The model under review builds one solid part; all positions refer to its coordinate system, in mm. A direction names the side the tool comes from. Coordinates: 2 decimals unless noted, no trailing zeros. Order: outer loops, then holes, each group sorted by start corner. A loop starts at its lowest first (then second) coordinate and runs counter-clockwise, first axis right, second up. Notation, with made-up numbers: (65.25, -32.5) -> (86.25, -32.5) arc R14 cw to (86.25, -26.5) -> close; hole circle Ø2 at (-18, 43). An arc over 180 degrees is marked (long way). Put each result on its own line as item: value.
from build123d import *

# Parameters (mm, degrees)
SKETCH1_W               = 12.7
SKETCH1_H               = 4.064
BOSS_EXTRUDE1_DEPTH     = 228.6
SKETCH2_W               = 3.429
SKETCH2_H               = 217.3732
CUT_EXTRUDE1_DEPTH      = 0.254
SKETCH3_W               = 0.508
SKETCH3_H               = 5.08
CUT_EXTRUDE2_DEPTH      = 229.724285103
MIRROR2_COPY_1_SKETCH_W = 0.508
MIRROR2_COPY_1_SKETCH_H = 5.08
MIRROR2_COPY_1_DEPTH    = 229.724285103
SKETCH4_W               = 3.175
SKETCH4_H               = 3.175
CUT_EXTRUDE3_DEPTH      = 229.724285103
CUT_EXTRUDE5_DEPTH      = 229.724285103
SKETCH6_W               = 6.80212
SKETCH6_H               = 6.80212
SKETCH6_R               = 1.70053
BOSS_EXTRUDE2_DEPTH     = 4.064
FILLET1_R               = 2.54


with BuildPart() as part:
    # Sketch1 → Boss-Extrude1 (new body)
    with BuildSketch(Plane.XY):
        Rectangle(SKETCH1_W, SKETCH1_H)
    extrude(amount=BOSS_EXTRUDE1_DEPTH)

    # Sketch2 → Cut-Extrude1 (cut)
    with BuildSketch(Plane(origin=(0, 2.032, 0), x_dir=(1, 0, 0), z_dir=(0, 1, 0))):
        with Locations((0, -114.3)):
            Rectangle(SKETCH2_W, SKETCH2_H)
    extrude(amount=-CUT_EXTRUDE1_DEPTH, mode=Mode.SUBTRACT)

    # Sketch3 → Cut-Extrude2 (cut, through all)
    with BuildSketch(Plane(origin=(0, 2.032, 0), x_dir=(1, 0, 0), z_dir=(0, 1, 0))):
        with Locations((-6.096, -226.06)):
            Rectangle(SKETCH3_W, SKETCH3_H)
    cut_extrude2 = extrude(amount=-CUT_EXTRUDE2_DEPTH, mode=Mode.SUBTRACT)

    # Mirror1: Cut-Extrude2 across plane
    add(cut_extrude2.mirror(Plane(origin=(0, 0, 114.3), x_dir=(1, 0, 0), z_dir=(0, 0, -1))), mode=Mode.SUBTRACT)

    # Mirror2: Cut-Extrude2 across plane
    add(cut_extrude2.mirror(Plane(origin=(0, 0, 0), x_dir=(0, 0, 1), z_dir=(1, 0, 0))), mode=Mode.SUBTRACT)

    # Mirror2 copy 1 sketch → Mirror2 copy 1 (cut, through all)
    with BuildSketch(Plane(origin=(0, 2.032, 228.6), x_dir=(-1, 0, 0), z_dir=(0, 1, 0))):
        with Locations((-6.096, -226.06)):
            Rectangle(MIRROR2_COPY_1_SKETCH_W, MIRROR2_COPY_1_SKETCH_H)
    extrude(amount=-MIRROR2_COPY_1_DEPTH, mode=Mode.SUBTRACT)

    # Sketch4 → Cut-Extrude3 (cut, through all)
    with BuildSketch(Plane(origin=(0, 2.032, 0), x_dir=(1, 0, 0), z_dir=(0, 1, 0))):
        with Locations((-4.2545, -227.0125)):
            Rectangle(SKETCH4_W, SKETCH4_H)
    extrude(amount=-CUT_EXTRUDE3_DEPTH, mode=Mode.SUBTRACT)

    # Sketch5 → Cut-Extrude5 (cut, through all)
    with BuildSketch(Plane(origin=(0, 2.032, 0), x_dir=(1, 0, 0), z_dir=(0, 1, 0))):
        Polygon((-6.35, -71.12), (-6.35, -152.4), (-6.35, -228.6), (6.35, -228.6), (6.35, -155.575), (6.35, -152.4), (6.35, -76.2), (-3.175, -76.2), (-3.175, -71.12), align=None)
    extrude(amount=-CUT_EXTRUDE5_DEPTH, mode=Mode.SUBTRACT)

    # Sketch6 → Boss-Extrude2 (add, through all)
    # profile 1 of 2: a face of its own
    with BuildSketch(Plane(origin=(0, 2.032, 0), x_dir=(1, 0, 0), z_dir=(0, 1, 0))):
        with Locations((9.75106, -38.1)):
            Rectangle(SKETCH6_W, SKETCH6_H)
        with Locations(Location((9.75106, -38.1, 0), (0, 0, 270))):
            Circle(SKETCH6_R, mode=Mode.SUBTRACT)
    # profile 2 of 2: a face of its own
    with BuildSketch(Plane(origin=(0, 2.032, 0), x_dir=(1, 0, 0), z_dir=(0, 1, 0))):
        with Locations((-9.75106, -38.1)):
            Rectangle(SKETCH6_W, SKETCH6_H)
        with Locations(Location((-9.75106, -38.1, 0), (0, 0, 90))):
            Circle(SKETCH6_R, mode=Mode.SUBTRACT)
    extrude(amount=-BOSS_EXTRUDE2_DEPTH)

    # Fillet1
    fillet1_edges = [part.edges().sort_by_distance(p)[0] for p in [
        (6.35, 0, 41.50106),
        (13.15212, 0, 41.50106),
        (13.15212, 0, 34.69894),
        (6.35, 0, 34.69894),
        (-6.35, 0, 34.69894),
        (-13.15212, 0, 34.69894),
        (-13.15212, 0, 41.50106),
        (-6.35, 0, 41.50106),
    ]]
    fillet(fillet1_edges, radius=FILLET1_R)


solid = part.part
Item 1: Consider section B-B on x = -0.5. Write out the cut boundary in (y, z).
Answers below:
outline: (-2.03, 0) -> (2.03, 0) -> (2.03, 5.61) -> (1.78, 5.61) -> (1.78, 76.2) -> (-2.03, 76.2) -> close
Item 2: Consider section A-A on z = 38.1. Write out the cut boundary in (x, y), and give its area (3 significant figures).
Answers below:
outline: (-13.15, -2.03) -> (-11.45, -2.03) -> (-11.45, 2.03) -> (-13.15, 2.03) -> close; (-8.05, -2.03) -> (8.05, -2.03) -> (8.05, 2.03) -> (1.71, 2.03) -> (1.71, 1.78) -> (-1.71, 1.78) -> (-1.71, 2.03) -> (-8.05, 2.03) -> close; (11.45, -2.03) -> (13.15, -2.03) -> (13.15, 2.03) -> (11.45, 2.03) -> close
area: 78.4 mm^2
Item 3: Consider section D-D on y = 0.45. Write out the cut boundary in (x, z) (3 decimals).
Answers below:
outline: (-13.152, 37.239) arc R2.54 ccw to (-10.612, 34.699) -> (-8.89, 34.699) arc R2.54 cw to (-6.35, 32.159) -> (-6.35, 5.08) -> (-5.842, 5.08) -> (-5.842, 0) -> (5.842, 0) -> (5.842, 5.08) -> (6.35, 5.08) -> (6.35, 32.159) arc R2.54 cw to (8.89, 34.699) -> (10.612, 34.699) arc R2.54 ccw to (13.152, 37.239) -> (13.152, 38.961) arc R2.54 ccw to (10.612, 41.501) -> (8.89, 41.501) arc R2.54 cw to (6.35, 44.041) -> (6.35, 76.2) -> (-3.175, 76.2) -> (-3.175, 71.12) -> (-6.35, 71.12) -> (-6.35, 44.041) arc R2.54 cw to (-8.89, 41.501) -> (-10.612, 41.501) arc R2.54 ccw to (-13.152, 38.961) -> close; hole circle Ø3.401 at (-9.751, 38.1); hole circle Ø3.401 at (9.751, 38.1)
Item 4: Consider section C-C on z = 24.5. Write out the cut boundary in (x, y), and give its area (3 significant figures).
Answers below:
outline: (-6.35, -2.03) -> (6.35, -2.03) -> (6.35, 2.03) -> (1.71, 2.03) -> (1.71, 1.78) -> (-1.71, 1.78) -> (-1.71, 2.03) -> (-6.35, 2.03) -> close
area: 50.7 mm^2
Item 5: For line 1 (X direction, y = 1.25, z = 38.1); line 2 (X direction, y = 1.45, z = 38.5); line 3 (X direction, y = 0.4, z = 49.5), list the stretches that pass through material, from the lowest coordinate up. Write a range as from..to.
Answers below:
line 1: -13.15..-11.45, -8.05..8.05, 11.45..13.15
line 2: -13.15..-11.4, -8.1..8.1, 11.4..13.15
line 3: -6.35..6.35
Item 6: Mouldability with a two-part tool opening along Z and no side actions: class faces 1 (the cylindrical face through (-9.1, 0.03, 36.53)), 2 (the flat face through (2, 0, 76.2)), 3 (the flat face through (0, 0, 0)) as +Z half, -Z half, draft (parallel to the pull), parting line (faces both ways), or undercut.
Answers below:
face 1: undercut
face 2: +Z half
face 3: -Z half
Item 7: For pin 1 Ø0.9 at (x, y) = (10, 1) entering from -Z; pin 2 Ø1 at (x, y) = (7.5, -1) entering from -Z; pin 3 Ø1.9 at (x, y) = (-10, -0.5) entering from +Z, all flat-tipped, find the tip position at first contact; note any pin that passes through.
Answers below:
pin 1: z = 34.7
pin 2: z = 33.86
pin 3: z = 41.5
Item 8: For faces 4 (the flat face through (-6.35, 0, 57)), 5 (the flat face through (10, 0, 34.699)), 6 (the flat face through (-6.35, 0, 18)), 7 (the flat face through (0, 1.778, 40)), 8 (the flat face through (6.35, 0, 60)), list the 3-axis set-ups (+Z, -Z, +X, -X, +Y, -Y) from which the entire face can be reached by the end or side of a thin tool; tool diameter is ignored.
Answers below:
face 4: +Z, -X, +Y, -Y
face 5: -Z, +X, +Y, -Y
face 6: -Z, -X, +Y, -Y
face 7: +Z, +Y
face 8: +Z, +X, +Y, -Y
